```python
from build123d import *

# Parameters (mm, degrees)
BOSS_EXTRUDE1_DEPTH = 0.2
BOSS_EXTRUDE2_DEPTH = 12.58
SKETCH1_4_W         = 149.48
SKETCH1_4_H         = 2
BOSS_EXTRUDE3_DEPTH = 15.58


with BuildPart() as part:
    # Sketch1 → Boss-Extrude1 (new body)
    with BuildSketch(Plane(origin=(0, 0, 0), x_dir=(1, 0, 0), z_dir=(0, 1, 0))):
        Polygon((-42.01, 19.39179677), (-101.494739838, 19.39179677), (-112.690598923, 0), (-109.845299462, -4.92820323), (-74.74, -4.92820323), (74.74, -4.92820323), (109.845299462, -4.92820323), (112.690598923, 0), (101.494739838, 19.39179677), (50.01, 19.39179677), (50.01, 21.39179677), (-42.01, 21.39179677), align=None)
    extrude(amount=BOSS_EXTRUDE1_DEPTH)

    # Sketch1<3> → Boss-Extrude2 (add)
    with BuildSketch(Plane(origin=(0, 0, 0), x_dir=(1, 0, 0), z_dir=(0, 1, 0))):
        Polygon((-115, 0), (-111, -6.92820323), (-74.74, -6.92820323), (-74.74, -4.92820323), (-109.845299462, -4.92820323), (-112.690598923, 0), (-101.494739838, 19.39179677), (-102.649440377, 21.39179677), align=None)
        Polygon((115, 0), (111, -6.92820323), (74.74, -6.92820323), (74.74, -4.92820323), (109.845299462, -4.92820323), (112.690598923, 0), (101.494739838, 19.39179677), (102.649440377, 21.39179677), align=None)
    extrude(amount=BOSS_EXTRUDE2_DEPTH)

    # Sketch1<4> → Boss-Extrude3 (add)
    with BuildSketch(Plane(origin=(0, 0, 0), x_dir=(1, 0, 0), z_dir=(0, 1, 0))):
        Polygon((-42.01, 21.39179677), (-102.649440377, 21.39179677), (-101.494739838, 19.39179677), (-42.01, 19.39179677), align=None)
        with Locations((0, -5.92820323)):
            Rectangle(SKETCH1_4_W, SKETCH1_4_H)
        Polygon((102.649440377, 21.39179677), (50.01, 21.39179677), (50.01, 19.39179677), (101.494739838, 19.39179677), align=None)
    extrude(amount=BOSS_EXTRUDE3_DEPTH)


solid = part.part
```
Work out the finished part from the listing and answer in its coordinate system (mm). A direction names the side the tool comes from. Round coordinates to 2 decimals unless told otherwise and drop trailing zeros. Write each loop counter-clockwise with the first axis right and the second up, starting at its lowest first coordinate (ties: lowest second). Pieces come first, ordered by that corner, then holes.
1) A cutting plane is placed at A-A on x = 63.5. Determine the outline of the cut face in (y, z), and give its area (3 significant figures).
2) Flat-ended cylindrical pins translate along their axes: P1, Ø8.5, axis at x = 98.5, z = -2.5, coming from the +Y side; P2, Ø1, axis at y = 9.5, z = -20.5, coming from the -X side; P3, Ø2, axis at y = 6, z = -20, coming from the +X side; P4, Ø8, axis at x = 74.5, z = -9, coming from the -Y side. Find the tip coordinate at first contact, or state that the pin passes through.
3) A cutting plane is placed at C-C on z = -2. Determine the outline of the cut face in (x, y).
4) Which of the six approach directions +Z, -Z, +X, -X, +Y, -Y give full straight-line access (tool end or side, diameter ignored) to faces 5 (the face through (-99.4, 12.58, 5.3)), 6 (the face through (-44, 8, -21.392)), 7 (the face through (-107.17, 6.3, -9.56))?
5) Determine the mould class of faces 1 (the face through (-111.248, 6.303, 2.499)), 2 (the face through (-108.738, 6.202, -10.846)), 3 (the face through (113.028, 6.202, 3.416)), 4 (the face through (99.4, 12.58, 5.3)) for opening direction Z: pulls with the +Z half, pulls with the -Z half, needs draft (parallel to the pull), parting line crosses it, or undercut.
6) Consider probe 1 along Z at (x, y) = (101.5, 1); probe 2 along Y at (x, z) = (42, -18.75); probe 3 along Z at (x, y) = (-31.5, 2). Determine where each line is inside the solid, lowest interval first.
7) A cutting plane is placed at D-D on x = 29. Determine the outline of the cut face in (y, z).
8) A cutting plane is placed at B-B on y = 10.5. Determine the outline of the cut face in (x, z).
Entries:
1. outline: (0, -21.39) - (15.58, -21.39) - (15.58, -19.39) - (0.2, -19.39) - (0.2, 4.93) - (15.58, 4.93) - (15.58, 6.93) - (0, 6.93) - close
1. area: 67.2 mm2
2. P1: stops at y = 0.2
2. P2: stops at x = -103.45
2. P3: stops at x = 104.03
2. P4: stops at y = 0
3. outline: (-113.85, 0) - (113.85, 0) - (113.85, 12.58) - (111.54, 12.58) - (111.54, 0.2) - (-111.54, 0.2) - (-111.54, 12.58) - (-113.85, 12.58) - close
4. face 5: +Z, -X, +Y
4. face 6: -Z, +X, -X, +Y, -Y
4. face 7: +Y
5. face 1: undercut
5. face 2: pulls with the -Z half
5. face 3: pulls with the +Z half
5. face 4: needs draft
6. probe 1: z = -21.39 to -19.38, 4.93 to 6.93
6. probe 2: y = 0 to 0.2
6. probe 3: z = 4.93 to 6.93
7. outline: (0, -21.39) - (0.2, -21.39) - (0.2, 4.93) - (15.58, 4.93) - (15.58, 6.93) - (0, 6.93) - close
8. outline: (-115, 0) - (-102.65, -21.39) - (-42.01, -21.39) - (-42.01, -19.39) - (-101.49, -19.39) - (-112.69, 0) - (-109.85, 4.93) - (109.85, 4.93) - (112.69, 0) - (101.49, -19.39) - (50.01, -19.39) - (50.01, -21.39) - (102.65, -21.39) - (115, 0) - (111, 6.93) - (-111, 6.93) - close
